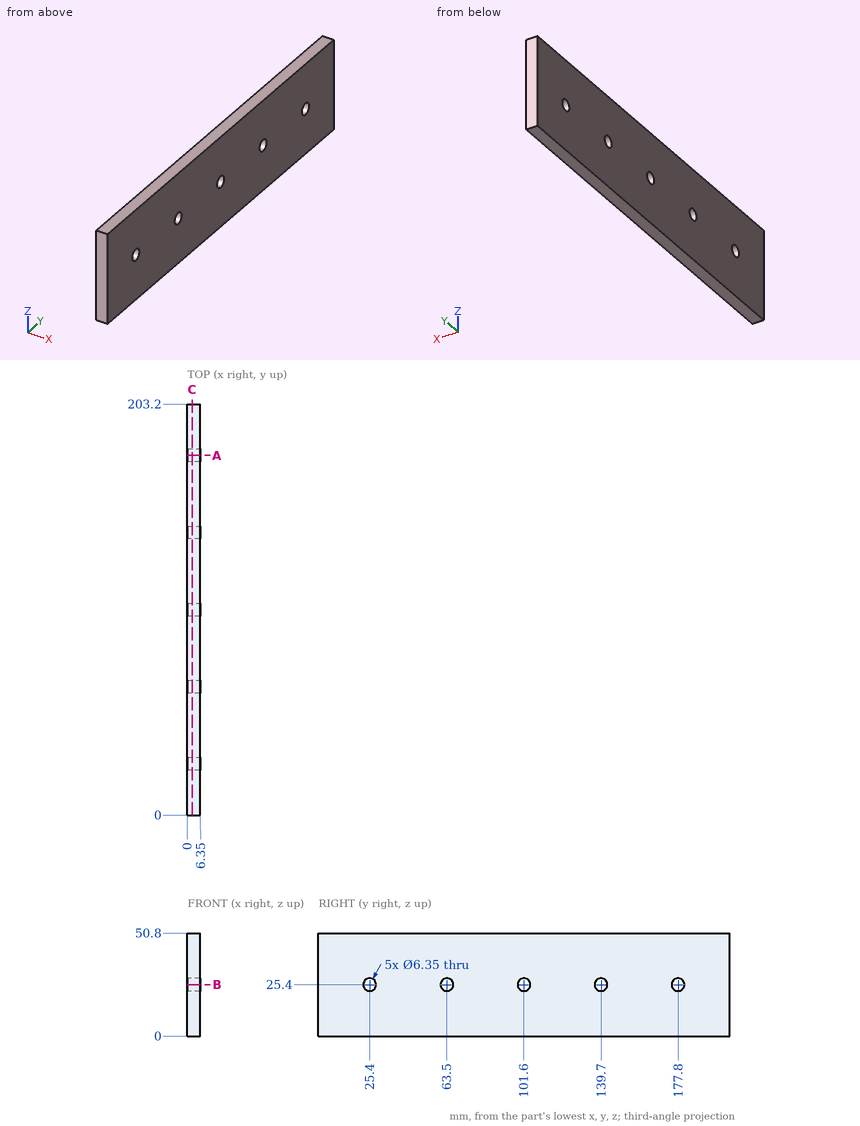
Print and shaded views of the part. All mm, measured from the part's lowest x, y and z. Coordinates: 2 decimals unless noted, no trailing zeros. Write each loop counter-clockwise with the first axis right and the second up, starting at its lowest first coordinate (ties: lowest second). Pieces come first, ordered by that corner, then holes.
(1) Drill centre lines: probe 1 along Y at (x, z) = (5, 25); probe 2 along Z at (x, y) = (3.75, 63.5) (3 decimals). Where is each one in solid material? Low to high.
(2) Cut at B-B, the plane z = 25.4. List the corners of the cut face in (x, y) (3 decimals), and give its area (3 significant figures).
(3) Cut at C-C, the plane x = 2.25. List the corners of the cut face in (y, z) (3 decimals).
(4) Flat gauge pin, fed straight in: pin 1 (3 mm diameter, centred on y = 134.5, z = 30, fed in from -X). Where does the tip first touch, or does it go through?
(5) Cut at A-A, the plane y = 177.8. List the corners of the cut face in (x, z) (3 decimals), and give its area (3 significant figures).
Geometry says:
1. probe 1: y = 0 to 22.25, 28.55 to 60.35, 66.65 to 98.45, 104.75 to 136.55, 142.85 to 174.65, 180.95 to 203.2
1. probe 2: z = 0 to 22.225, 28.575 to 50.8
2. outline: (0, 0) - (6.35, 0) - (6.35, 22.225) - (0, 22.225) - close; (0, 28.575) - (6.35, 28.575) - (6.35, 60.325) - (0, 60.325) - close; (0, 66.675) - (6.35, 66.675) - (6.35, 98.425) - (0, 98.425) - close; (0, 104.775) - (6.35, 104.775) - (6.35, 136.525) - (0, 136.525) - close; (0, 142.875) - (6.35, 142.875) - (6.35, 174.625) - (0, 174.625) - close; (0, 180.975) - (6.35, 180.975) - (6.35, 203.2) - (0, 203.2) - close
2. area: 1,090 mm2
3. outline: (0, 0) - (203.2, 0) - (203.2, 50.8) - (0, 50.8) - close; hole circle Ø6.35 at (25.4, 25.4); hole circle Ø6.35 at (63.5, 25.4); hole circle Ø6.35 at (101.6, 25.4); hole circle Ø6.35 at (139.7, 25.4); hole circle Ø6.35 at (177.8, 25.4)
4. pin 1: stops at x = 0
5. outline: (0, 0) - (6.35, 0) - (6.35, 22.225) - (0, 22.225) - close; (0, 28.575) - (6.35, 28.575) - (6.35, 50.8) - (0, 50.8) - close
5. area: 282 mm2
